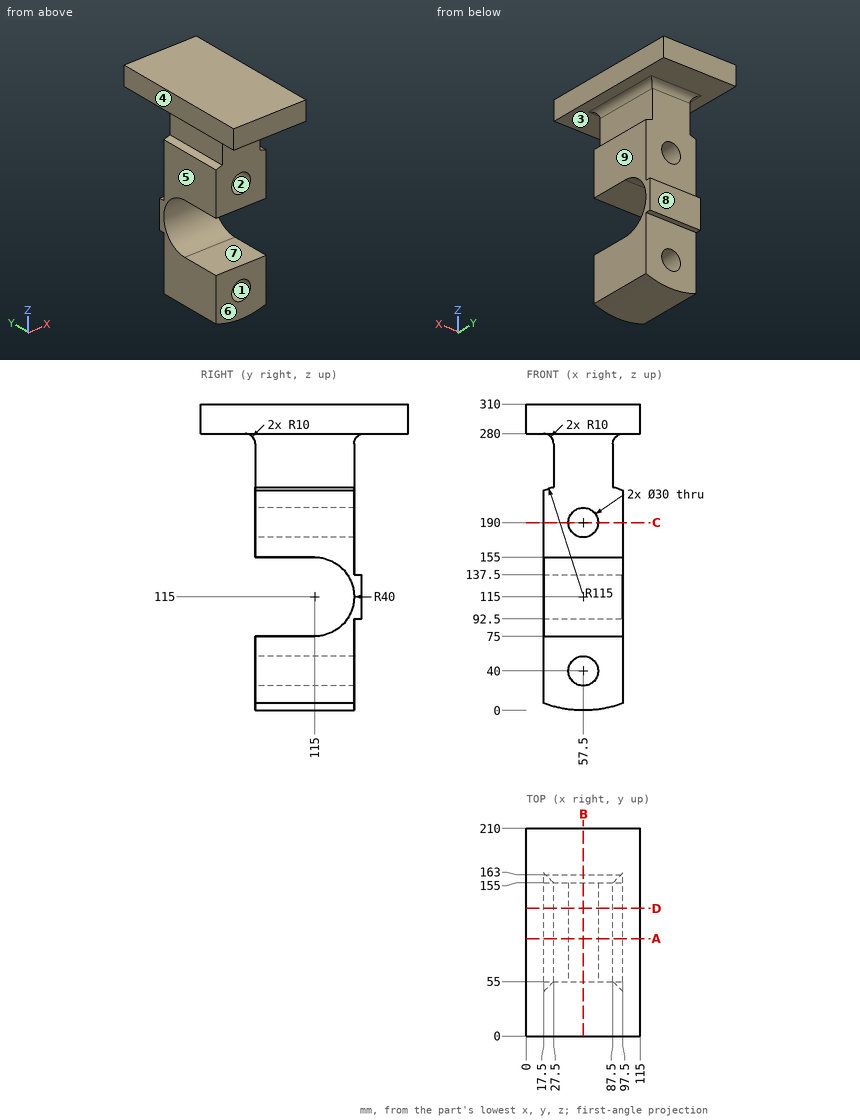
Design review of the part shown in the three views and the two pictorial views. Dimensions are in mm from the part's minimum x, y and z. A direction names the side the tool comes from. Coordinates: 2 decimals unless noted, no trailing zeros. Order: outer loops, then holes, each group sorted by start corner. A loop starts at its lowest first (then second) coordinate and runs counter-clockwise, first axis right, second up. Notation, with made-up numbers: (39, 79.5) - (47, 79.5) arc R27 ccw to (47, 109.5) - close; hole circle Ø7 at (-34, 30). An arc over 180 degrees is marked (long way). One line per question, with ' | ' between items.
Q1. For the marked faces 5, 6, 7, 8 and 9, list the 3-axis set-ups (+Z, -Z, +X, -X, +Y, -Y) from which the entire face can be reached by the end or side of a thin tool; tool diameter is ignored.
Answer key:
face 5: -Z, -X, +Y, -Y | face 6: -Z, +X, -X, -Y | face 7: +X, -X, -Y | face 8: -Z, +X, -X, +Y | face 9: -Z, +X, +Y, -Y
Q2. Consider section A-A, the plane y = 98.5. Give the boundary of the cut face in (x, z).
Answer key:
outline: (0, 280) - (17.5, 280) arc R10 cw to (27.5, 270) - (27.5, 226.02) arc R115 ccw to (17.5, 222.82) - (17.5, 155) - (97.5, 155) - (97.5, 222.82) arc R115 ccw to (87.5, 226.02) - (87.5, 270) arc R10 cw to (97.5, 280) - (115, 280) - (115, 310) - (0, 310) - close; (17.5, 7.18) arc R115 ccw to (97.5, 7.18) - (97.5, 75) - (17.5, 75) - close; hole circle Ø30 at (57.5, 40); hole circle Ø30 at (57.5, 190)
Q3. To check wall thickness, follow line 1 along X through (y, z) = (132, 40); line 2 along Z through (x, y) = (57, 112); line 3 along Z through (x, y) = (100, 53). State the ranges of each line that lie inside material, in increasing order.
Answer key:
line 1: x = 17.5 to 42.5, 72.5 to 97.5 | line 2: z = 0 to 25.01, 54.99 to 75, 155 to 175.01, 204.99 to 310 | line 3: z = 280 to 310
Q4. The part is to be moulded in two halves that separate along Z. For the marked faces 1, 2, 3 and 4, say which applies: +Z half, -Z half, draft (parallel to the pull), parting line (faces both ways), or undercut.
Answer key:
face 1: undercut | face 2: undercut | face 3: -Z half | face 4: draft
Q5. Clearance check with flat-ended pins moving along their axes: pin 1 Ø13 at (y, z) = (104.5, 256) entering from -X; pin 2 Ø13.5 at (x, z) = (75.5, 125.5) entering from +Y; pin 3 Ø24 at (x, z) = (61, 194.5) entering from +Y. State where each tip first meets the part, or that it passes through.
Answer key:
pin 1: stops at x = 27.5 | pin 2: stops at y = 163 | pin 3: stops at y = 155
Q6. Consider section C-C, the plane z = 190. Give the boundary of the cut face in (x, y), then the cut area to 3 significant figures.
Answer key:
outline: (17.5, 55) - (42.5, 55) - (42.5, 155) - (17.5, 155) - close; (72.5, 55) - (97.5, 55) - (97.5, 155) - (72.5, 155) - close | area: 5,000 mm2
Q7. Consider section B-B, the plane x = 57.5. Give the boundary of the cut face in (y, z).
Answer key:
outline: (0, 280) - (45, 280) arc R10 cw to (55, 270) - (55, 205) - (155, 205) - (155, 270) arc R10 cw to (165, 280) - (210, 280) - (210, 310) - (0, 310) - close; (55, 0) - (155, 0) - (155, 25) - (55, 25) - close; (55, 55) - (155, 55) - (155, 92.5) - (163, 92.5) - (163, 137.5) - (155, 137.5) - (155, 175) - (55, 175) - (55, 155) - (115, 155) arc R40 cw to (115, 75) - (55, 75) - close
Q8. Consider section D-D, the plane y = 129. Give the boundary of the cut face in (x, z), then the cut area to 3 significant figures.
Answer key:
outline: (0, 280) - (17.5, 280) arc R10 cw to (27.5, 270) - (27.5, 226.02) arc R115 ccw to (17.5, 222.82) - (17.5, 152.47) - (97.5, 152.47) - (97.5, 222.82) arc R115 ccw to (87.5, 226.02) - (87.5, 270) arc R10 cw to (97.5, 280) - (115, 280) - (115, 310) - (0, 310) - close; (17.5, 7.18) arc R115 ccw to (97.5, 7.18) - (97.5, 77.53) - (17.5, 77.53) - close; hole circle Ø30 at (57.5, 40); hole circle Ø30 at (57.5, 190) | area: 17,200 mm2
